The model under review builds one solid part; all positions refer to its coordinate system, in mm. A direction names the side the tool comes from. Coordinates: 2 decimals unless noted, no trailing zeros. Write each loop counter-clockwise with the first axis right and the second up, starting at its lowest first coordinate (ties: lowest second). Pieces come first, ordered by that corner, then holes. Notation, with made-up numbers: (-7, 58.25) - (26, 58.25) arc R16 ccw to (26, 64.25) - close; hole circle Ø1 at (5.5, -20.75). An arc over 180 degrees is marked (long way). Put each result on its own line as item: value.
from build123d import *

# Parameters (mm, degrees)
SKETCH2_W                = 150
SKETCH2_H                = 12.5
BOSS_EXTRUDE1_DEPTH      = 5
BOSS_EXTRUDE2_DEPTH      = 10
BOSS_EXTRUDE2_DEPTH_BACK = 10
SKETCH3_R                = 2
FILLET1_R                = 10
SKETCH4_R                = 1
CUT_EXTRUDE1_DEPTH       = 80.711981534
CUT_EXTRUDE2_START       = -20
SKETCH5_W                = 1
SKETCH5_H                = 4
CUT_EXTRUDE2_DEPTH       = 20
SKETCH6_W                = 120
SKETCH6_H                = 1.5
CUT_EXTRUDE3_DEPTH       = 2


with BuildPart() as part:
    # Sketch2 → Boss-Extrude1 (new body)
    with BuildSketch(Plane(origin=(0, 0, 0), x_dir=(1, 0, 0), z_dir=(0, 1, 0))):
        Rectangle(SKETCH2_W, SKETCH2_H)
    extrude(amount=BOSS_EXTRUDE1_DEPTH)

    # Sketch3 → Boss-Extrude2 (add, two sides: drawn at the far end of the back side and taken through both)
    with BuildSketch(Plane.XY.offset(-BOSS_EXTRUDE2_DEPTH_BACK)):
        with Locations((-75, 2.5)):
            Circle(SKETCH3_R)
    extrude(amount=BOSS_EXTRUDE2_DEPTH + BOSS_EXTRUDE2_DEPTH_BACK)

    # Fillet1
    # the kernel refuses this fillet: 10 mm, written as the material it adds along each edge
    with BuildSketch(Plane(origin=(-75, 4.5, 6.25), x_dir=(-5.0590642785823295e-12, 1.0, 0), z_dir=(0, 0, -1))) as fillet1_piece_1:
        with BuildLine():
            CenterArc((8.05, -6.557247898), FILLET1_R, 139.025369771, 7.851690022)
            Line((-0.325, -1.09287465), (-0.4925, -0.983587185))
            ThreePointArc((-0.4925, -0.983587185), (-0.274673944, -0.513078941), (-0.2, 0))
            Line((-0.2, 0), (0, 0.2))
            ThreePointArc((0, 0.2), (0.25, 0.2), (0.349, 0.131144958))
            Line((0.349, 0.131144958), (0.5, 0))
        make_face()
    extrude(amount=6.25)
    with BuildSketch(Plane(origin=(-75, 0.5, 6.25), x_dir=(-5.059064278582354e-12, -1.0, 0), z_dir=(0, 0, -1)), Plane(origin=(-75, 4.5, -6.25), x_dir=(-5.0590642785823295e-12, 1.0, 0), z_dir=(0, 0, 1))) as fillet1_piece_2:
        with BuildLine():
            CenterArc((8.05, 6.557247898), FILLET1_R, 213.122940208, 7.851690022)
            Line((-0.325, 1.09287465), (-0.4925, 0.983587185))
            ThreePointArc((-0.4925, 0.983587185), (-0.274673944, 0.513078941), (-0.2, 0))
            Line((-0.2, 0), (0, -0.2))
            ThreePointArc((0, -0.2), (0.25, -0.2), (0.349, -0.131144958))
            Line((0.349, -0.131144958), (0.5, 0))
        make_face()
    extrude(amount=6.25)
    with BuildSketch(Plane(origin=(-75, 0.5, -6.25), x_dir=(-0.9585144756337048, 0.2850438562759136, 0), z_dir=(0, 0, 1))) as fillet1_piece_3:
        with BuildLine():
            CenterArc((3.990613988, 9.585144756), FILLET1_R, 245.586839874, 7.851690022)
            Line((-0.142521928, 0.479257238), (-0.225184646, 0.297139487))
            ThreePointArc((-0.225184646, 0.297139487), (-0.262963859, 0.182619848), (-0.191702895, -0.057008771))
            Line((-0.191702895, -0.057008771), (0.057008771, -0.191702895))
            ThreePointArc((0.057008771, -0.191702895), (0.570087713, -0.117028951), (1.083166654, -0.191702895))
            Line((1.083166654, -0.191702895), (1.140175425, 0))
        make_face()
    extrude(amount=6.25)

    # Sketch4 → Cut-Extrude1 (cut, through all)
    with BuildSketch(Plane.XY.offset(10)):
        with Locations((-75, 2.5)):
            Circle(SKETCH4_R)
    extrude(amount=-CUT_EXTRUDE1_DEPTH, mode=Mode.SUBTRACT)

    # Sketch5 → Cut-Extrude2 (cut)
    with BuildSketch(Plane.XY.offset(10).offset(CUT_EXTRUDE2_START)):
        with Locations((-75, 2.5)):
            Rectangle(SKETCH5_W, SKETCH5_H)
    cut_extrude2 = extrude(amount=CUT_EXTRUDE2_DEPTH, mode=Mode.SUBTRACT)

    # Mirror3: Cut-Extrude2 across plane
    add(cut_extrude2.mirror(Plane.XY), mode=Mode.SUBTRACT)

    # Sketch6 → Cut-Extrude3 (cut)
    with BuildSketch(Plane.XY.offset(6.25)):
        with Locations((15, 2.5)):
            Rectangle(SKETCH6_W, SKETCH6_H)
    cut_extrude3 = extrude(amount=-CUT_EXTRUDE3_DEPTH, mode=Mode.SUBTRACT)

    # Mirror4: Cut-Extrude3 across plane
    add(cut_extrude3.mirror(Plane.XY), mode=Mode.SUBTRACT)


solid = part.part
1. Machinability: for faces 1 (the cylindrical face through (-73, 2.5, -8.2)), 2 (the cylindrical face through (-73, 2.5, 8.1)), 3 (the flat face through (-1, 5, 0)), which of the approach directions +Z, -Z, +X, -X, +Y, -Y give a long, thin tool a straight path to every point of the face, cutting with its end or side? Answer none if there is none.
Determined:
face 1: -Z, +X
face 2: +Z, +X
face 3: +Z, -Z, +X, -X, +Y
2. For pin 1 Ø6 at (x, z) = (-11.5, 7.5) entering from -Y; pin 2 Ø1.2 at (x, y) = (36, 2.5) entering from -Z; pin 3 Ø0.9 at (y, z) = (1, 2.5) entering from -X; pin 4 Ø3 at (x, y) = (41.5, 2.5) entering from -Z, all flat-tipped, find the tip position at first contact; note any pin that passes through.
Determined:
pin 1: stops at y = 0
pin 2: stops at z = -4.25
pin 3: stops at x = -76.7
pin 4: stops at z = -6.25
3. To check wall thickness, follow probe 1 along Z at (x, y) = (26.5, 1.6); probe 2 along X at (y, z) = (3.05, 6); probe 3 along Z at (x, y) = (-15, 1.95). State the ranges of each line that lie inside material, in increasing order.
Determined:
probe 1: z = -6.25 to 6.25
probe 2: x = -76.92 to -75.84, -74.16 to -45
probe 3: z = -4.25 to 4.25
4. Consider section B-B on x = 27.5. State the section outline as (y, z) points.
Determined:
outline: (0, -6.25) - (1.75, -6.25) - (1.75, -4.25) - (3.25, -4.25) - (3.25, -6.25) - (5, -6.25) - (5, 6.25) - (3.25, 6.25) - (3.25, 4.25) - (1.75, 4.25) - (1.75, 6.25) - (0, 6.25) - close
5. Consider section A-A on z = -7.5. State the section outline as (x, y) points.
Determined:
outline: (-75.5, 0.56) - (-75.5, 1.63) arc R1 cw to (-75.5, 3.37) - (-75.5, 4.44) arc R2 ccw to start; (-74.5, 0.56) arc R2 ccw to (-74.5, 4.44) - (-74.5, 3.37) arc R1 cw to (-74.5, 1.63) - close
